Geometry check sheet. Reference: drawing and pictorial views, mm from the part's lowest x, y, z. Round coordinates to 2 decimals unless told otherwise and drop trailing zeros. Write each loop counter-clockwise with the first axis right and the second up, starting at its lowest first coordinate (ties: lowest second). Pieces come first, ordered by that corner, then holes. Notation, with made-up numbers: M 8.25,30 L 59.25,30 A37 cw 59.25,68 Z; hole C 39,16.25 d3. An arc over 180 degrees is marked long. Put each result on its own line as item: value. Start each with the question number.
(1) Section check A-A on x = 12. Record the cut outline in (y, z), then the cut area to 3 significant figures.
(2) Mould release check, pull along Y, two halves, no side actions. Record for the marked faces 1 and 2: pulls with the +Y half, pulls with the -Y half, needs draft (parallel to the pull), parting line crosses it, or undercut.
(3) Material ranges on probe 1 along Y at (x, z) = (12, 2.5); probe 2 along X at (y, z) = (22, 7.75); probe 3 along Y at (x, z) = (10, 9.25), recorded low to high.
(4) Section check C-C on z = 9. Record the cut outline in (x, y).
(5) Gauge pin test, flat ends, axial feed: pin 1 (1.5 mm diameter, centred on x = 18.5, z = 1, fed in from +Y); pin 2 (4 mm diameter, centred on y = 4, z = 3, fed in from -X); pin 3 (5 mm diameter, centred on y = 4.5, z = 7.5, fed in from -X). Record the tip position at first contact, or that the pin passes through.
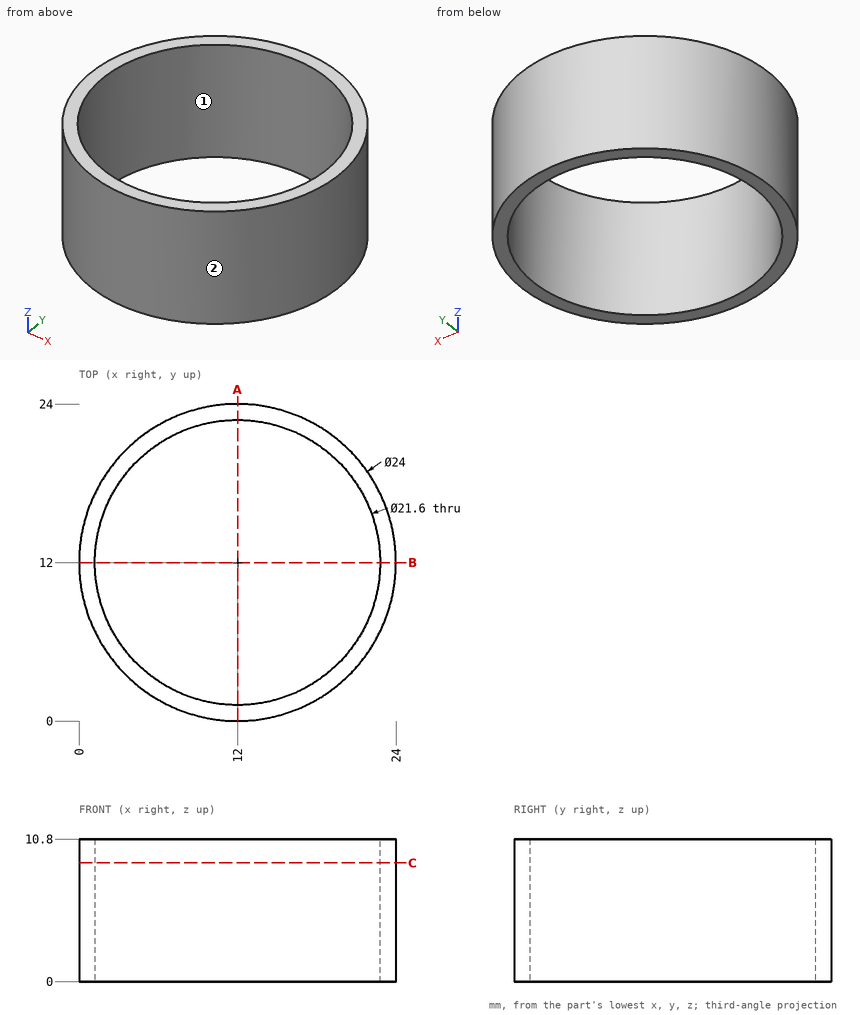
Answers follow:
1. outline: M 0,0 L 1.2,0 L 1.2,10.8 L 0,10.8 Z; M 22.8,0 L 24,0 L 24,10.8 L 22.8,10.8 Z
1. area: 25.9 mm^2
2. face 1: undercut
2. face 2: parting line crosses it
3. probe 1: y = 0 to 1.2, 22.8 to 24
3. probe 2: x = 5.37 to 7.92, 16.08 to 18.63
3. probe 3: y = 0.17 to 1.39, 22.61 to 23.83
4. outline: C 12,12 d24; hole C 12,12 d21.6
5. pin 1: stops at y = 22.53
5. pin 2: stops at x = 1.61
5. pin 3: stops at x = 1.09
